Study the drawing (mm; zero at the part's minimum x, y, z) and answer. Coordinates: 2 decimals unless noted, no trailing zeros. Write each loop counter-clockwise with the first axis right and the second up, starting at its lowest first coordinate (ties: lowest second). Pieces come first, ordered by that corner, then holes. Notation, with made-up numbers: (35, 1.5) -> (50, 1.5) arc R21 cw to (50, 7.5) -> close; hole circle Ø4 at (-34, 54). An arc over 180 degrees is marked (long way). Answer in a Markdown table with one row per item. Add a question column.
Item 1: Section A-A on z = 22 is taken. Write down the section's boundary in (x, y).
Item 2: For a pull along X with two mould halves and no side action, classify the marked faces 1, 2 and 3 as +X half, -X half, draft (parallel to the pull), parting line (faces both ways), or undercut.
Item 3: Section B-B on x = 118 is taken. Write down the section's boundary in (y, z).
Item 4: Straight lines are drawn through the part: line 1 (X direction, y = 34, z = 42); line 2 (X direction, y = 60, z = 52); line 3 (Z direction, x = 115.5, y = 30) (1 decimal). For each, find the intervals that lie inside material, in ascending order. Write a range as from..to.
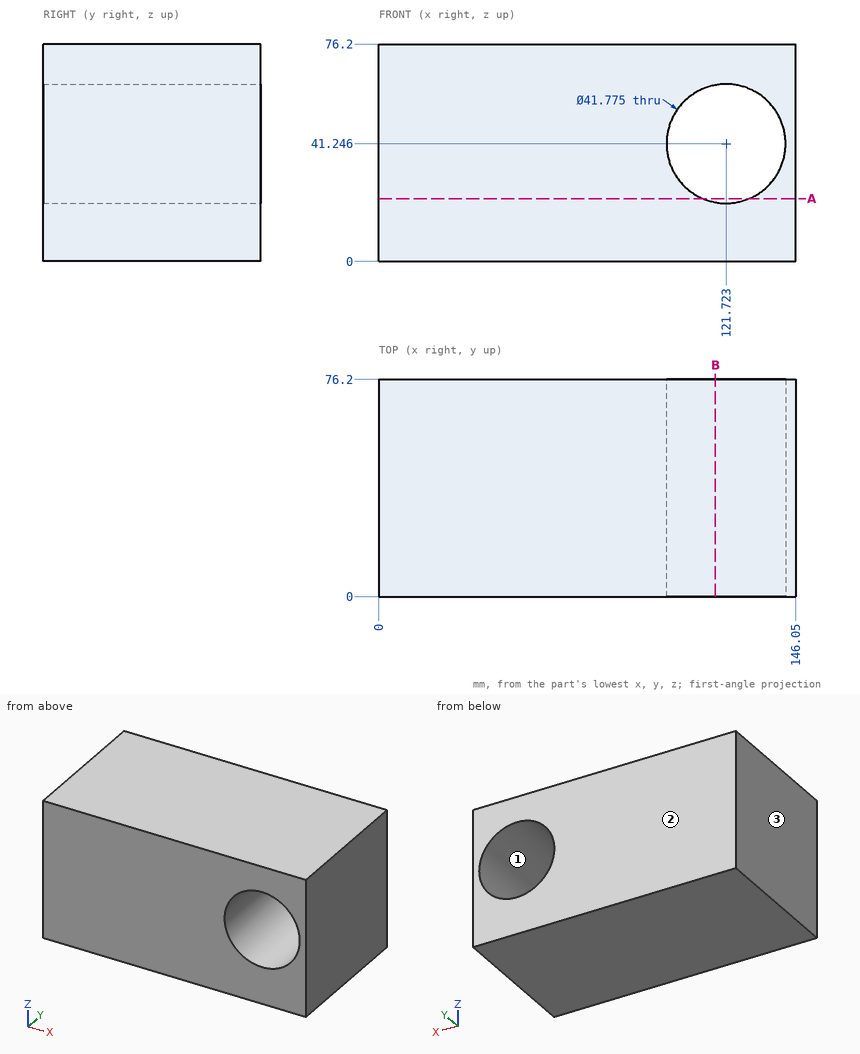
Results below:
| question | item | result |
|---|---|---|
| 1 | outline | (0, 0) -> (113.61, 0) -> (113.61, 76.2) -> (0, 76.2) -> close; (129.84, 0) -> (146.05, 0) -> (146.05, 76.2) -> (129.84, 76.2) -> close |
| 2 | face 1 | undercut |
| 2 | face 2 | draft |
| 2 | face 3 | -X half |
| 3 | outline | (0, 0) -> (76.2, 0) -> (76.2, 20.69) -> (0, 20.69) -> close; (0, 61.8) -> (76.2, 61.8) -> (76.2, 76.2) -> (0, 76.2) -> close |
| 4 | line 1 | x = 0..100.85, 142.6..146.05 |
| 4 | line 2 | x = 0..103.82, 139.63..146.05 |
| 4 | line 3 | z = 0..21.3, 61.2..76.2 |
